```python
from build123d import *

# Parameters (mm, degrees)
SKETCH1_W                 = 42.3
SKETCH1_H                 = 42.3
BOSS_EXTRUDE1_DEPTH       = 39.5
SKETCH2_R                 = 11
BOSS_EXTRUDE2_DEPTH       = 2
FILLET1_SIZE              = 6.35
F_4_0MM_DOWEL_HOLE1_D     = 4
F_4_0MM_DOWEL_HOLE1_DEPTH = 4.572
F_4_0MM_DOWEL_HOLE1_TIP   = 1.201721238
SKETCH6_R                 = 4
CUT_EXTRUDE1_DEPTH        = 37
SKETCH7_W                 = 16
SKETCH7_H                 = 9.6
BOSS_EXTRUDE3_DEPTH       = 7


with BuildPart() as part:
    # Sketch1 → Boss-Extrude1 (new body)
    with BuildSketch(Plane(origin=(0, 0, 0), x_dir=(1, 0, 0), z_dir=(0, 1, 0))):
        with Locations((6.409090909, -3.738636364)):
            Rectangle(SKETCH1_W, SKETCH1_H)
    extrude(amount=BOSS_EXTRUDE1_DEPTH)

    # Sketch2 → Boss-Extrude2 (add)
    with BuildSketch(Plane(origin=(0, 39.5, 0), x_dir=(1, 0, 0), z_dir=(0, 1, 0))):
        with Locations(Location((6.409090909, -3.738636364, 0), (0, 0, 270))):
            Circle(SKETCH2_R)
    extrude(amount=BOSS_EXTRUDE2_DEPTH)

    # Fillet1
    # a fillet whose section is not a circle: 6.35 mm, written as the material it takes off along each edge
    with BuildSketch(Plane(origin=(-14.740909091, -15.875, -17.411363636), x_dir=(1, 0, 0), z_dir=(0, 1, 0)), Plane(origin=(-14.740909091, -15.875, 24.888636364), x_dir=(0, 0, -1), z_dir=(0, 1, 0))) as fillet1_piece_1:
        with BuildLine():
            Bezier((FILLET1_SIZE, 0), (0, 0), (0, -FILLET1_SIZE), weights=[1, 0.449012806, 1])
            Line((0, -FILLET1_SIZE), (0, 0))
            Line((0, 0), (FILLET1_SIZE, 0))
        make_face()
    extrude(amount=71.25, mode=Mode.SUBTRACT)
    with BuildSketch(Plane(origin=(27.559090909, -15.875, -17.411363636), x_dir=(-1, 0, 0), z_dir=(0, 1, 0)), Plane(origin=(27.559090909, -15.875, 24.888636364), x_dir=(0, 0, -1), z_dir=(0, 1, 0))) as fillet1_piece_2:
        with BuildLine():
            Bezier((FILLET1_SIZE, 0), (0, 0), (0, FILLET1_SIZE), weights=[1, 0.449012806, 1])
            Line((0, FILLET1_SIZE), (0, 0))
            Line((0, 0), (FILLET1_SIZE, 0))
        make_face()
    extrude(amount=71.25, mode=Mode.SUBTRACT)

    # Ø4.0mm Dowel Hole1
    with Locations(Plane(origin=(0, 39.5, 0), x_dir=(1, 0, 0), z_dir=(0, 1, 0))):
        with Locations((-9.092111006, 11.76136359), (21.907888994, 11.76136359), (21.910292824, -19.238636317), (-9.089707176, -19.23863641)):
            Hole(F_4_0MM_DOWEL_HOLE1_D / 2, depth=F_4_0MM_DOWEL_HOLE1_DEPTH)
            with Locations((0, 0, -(F_4_0MM_DOWEL_HOLE1_DEPTH + F_4_0MM_DOWEL_HOLE1_TIP / 2))):  # 118° drill point
                Cone(0, F_4_0MM_DOWEL_HOLE1_D / 2, F_4_0MM_DOWEL_HOLE1_TIP, mode=Mode.SUBTRACT)

    # Sketch6 → Cut-Extrude1 (cut)
    with BuildSketch(Plane(origin=(0, 41.5, 0), x_dir=(1, 0, 0), z_dir=(0, 1, 0))):
        with Locations(Location((6.409090909, -3.738636364, 0), (0, 0, 270))):
            Circle(SKETCH6_R)
    extrude(amount=-CUT_EXTRUDE1_DEPTH, mode=Mode.SUBTRACT)

    # Sketch7 → Boss-Extrude3 (add)
    with BuildSketch(Plane(origin=(27.559090909, 0, 0), x_dir=(0, 0, -1), z_dir=(1, 0, 0))):
        with Locations((-3.15108899, 4.8)):
            Rectangle(SKETCH7_W, SKETCH7_H)
    extrude(amount=BOSS_EXTRUDE3_DEPTH)


solid = part.part
```
CAD build for the part. Positions are in the model's coordinates, mm. A direction names the side the tool comes from. Coordinates: 2 decimals unless noted, no trailing zeros. Write each loop counter-clockwise with the first axis right and the second up, starting at its lowest first coordinate (ties: lowest second). Pieces come first, ordered by that corner, then holes. Notation, with made-up numbers: (72, 72) -> (117, 72) arc R21 ccw to (117, 108) -> close; hole circle Ø10 at (88.25, -15.5). An arc over 180 degrees is marked (long way). Return JSON: item names as keys, results as strings. Group by question number.
Q1. Flat gauge pins, fed straight in: pin 1 (2.5 mm diameter, centred on x = -9.09, z = 19.24, fed in from -Y); pin 2 (5.5 mm diameter, centred on x = 32.5, y = 3.5, fed in from -Z); pin 3 (1 mm diameter, centred on x = -7.5, z = 0, fed in from +Y); pin 4 (2 mm diameter, centred on x = 30.5, z = 1, fed in from +Y). Where does each tip first touch, or does it go through?
Q2. Cut at D-D, the plane x = 31.5. Give the cut face in (y, z).
Q3. Pull direction X, two halves, no side cores. Call faces 4 (the face through (-8.7, 37.2, -9.8)), 5 (the face through (-14.741, 19, 4)), 6 (the face through (-10.16, 37.18, 17.55)), 7 (the face through (31, 5, 11.151)): released by +X, released by -X, zero draft, split by the parting line, or undercut.
Q4. Cut at B-B, the plane x = -0.5. Give the cut face in (y, z), then the cut area to 3 significant figures.
Q5. Cut at C-C, the plane z = -8.5. Give the cut face in (x, y).
Q6. Drill centre lines: line 1 (Y direction, x = 22, z = 7.5); line 2 (X direction, y = 11.5, z = 11); line 3 (Y direction, x = 8, z = 0.5). Where is each one in solid material? Low to high.
Q7. Cut at A-A, the plane z = 12.5. Give the cut face in (x, y).
Q8. Which spindle directions (+Z, -Z, +X, -X, +Y, -Y) get a long thin tool onto all of the face, cutting with end or side? Do faces 1 (the face through (2.86, 23.26, 5.58)), 2 (the face through (31, 5, -4.849)), 3 (the face through (31, 9.6, 3)). Say none if no direction does.
Returned:
{
 "1": {"pin 1": "stops at y = 0", "pin 2": "stops at z = -4.85", "pin 3": "stops at y = 39.5", "pin 4": "stops at y = 9.6"},
 "2": {"outline": "(0, -4.85) -> (9.6, -4.85) -> (9.6, 11.15) -> (0, 11.15) -> close"},
 "3": {"face 4": "undercut", "face 5": "released by -X", "face 6": "undercut", "face 7": "zero draft"},
 "4": {"outline": "(0, -17.41) -> (39.5, -17.41) -> (39.5, -4.82) -> (41.5, -4.82) -> (41.5, 12.3) -> (39.5, 12.3) -> (39.5, 24.89) -> (0, 24.89) -> close", "area": "1,710 mm2"},
 "5": {"outline": "(-14.74, 0) -> (27.56, 0) -> (27.56, 39.5) -> (-14.74, 39.5) -> close"},
 "6": {"line 1": "y = 0 to 39.5", "line 2": "x = -14.74 to 27.56", "line 3": "y = 0 to 4.5"},
 "7": {"outline": "(-14.74, 0) -> (27.56, 0) -> (27.56, 39.5) -> (13.06, 39.5) -> (13.06, 41.5) -> (-0.24, 41.5) -> (-0.24, 39.5) -> (-14.74, 39.5) -> close"},
 "8": {"face 1": "+Y", "face 2": "-Z, +X, +Y, -Y", "face 3": "+Z, -Z, +X, +Y"}
}
